Read the model definition and answer for the solid it produces. Units are mm, in the model's axes. Face numbers are marked on the shaded views. A direction names the side the tool comes from. Coordinates: 2 decimals unless noted, no trailing zeros. Write each loop counter-clockwise with the first axis right and the second up, starting at its lowest first coordinate (ties: lowest second). Pieces come first, ordered by that corner, then holes. Notation, with made-up numbers: (68.25, 57) -> (90.25, 57) arc R20 cw to (90.25, 84) -> close; hole circle Ø9 at (-0.5, -6). An arc over 180 degrees is marked (long way). Answer as a JSON object with one key per item and string values. Group by question number.
(1) Which of the six approach directions +Z, -Z, +X, -X, +Y, -Y give full straight-line access (tool end or side, diameter ignored) to the marked faces 1 and 2?
(2) A flat-ended cylindrical pin translates along its axis: P1, Ø7.5, axis at x = 0, y = 52.34, coming from the +Z side. Find the tip coordinate at first contact, or state that the pin passes through.
(3) For a pull along Z with two mould halves and no side action, classify the marked faces 3, 4 and 5 as +Z half, -Z half, draft (parallel to the pull), parting line (faces both ways), or undercut.
(4) Find section D-D (x = 1). Count the separate pieces of the cut face and the enclosed holes in it, then the cut area to 3 significant figures.
(5) Straight lines are drawn through the part: L1, parallel to Z at x = 1, y = -45.5 (3 decimals); L2, parallel to Y at x = 0, z = 11.3. For each, find the intervals that lie inside material, in ascending order.
(6) Find section A-A (x = -5.75). Give the vertices of the cut face in (y, z) (3 decimals).
(7) Find section C-C (z = -3.5). Give the vertices of the cut face in (x, y) (3 decimals).
(8) Find section B-B (y = 37.5). Give the vertices of the cut face in (x, z) (3 decimals), then the cut area to 3 significant figures.
from build123d import *

# Parameters (mm, degrees)
SKETCH1_W           = 25.4
SKETCH1_H           = 25.4
SKETCH1_W_2         = 19.05
SKETCH1_H_2         = 19.05
BOSS_EXTRUDE1_DEPTH = 82.931
CUT_EXTRUDE1_DEPTH  = 88.658432344
SKETCH3_R           = 3.22238806
CUT_EXTRUDE2_DEPTH  = 88.658432344


with BuildPart() as part:
    # Sketch1 → Boss-Extrude1 (new, symmetric)
    with BuildSketch(Plane(origin=(0, 0, 0), x_dir=(1, 0, 0), z_dir=(0, 1, 0))):
        Rectangle(SKETCH1_W, SKETCH1_H)
        Rectangle(SKETCH1_W_2, SKETCH1_H_2, mode=Mode.SUBTRACT)
    extrude(amount=BOSS_EXTRUDE1_DEPTH, both=True)

    # Sketch2 → Cut-Extrude1 (cut, through all)
    with BuildSketch(Plane(origin=(12.7, 0, 0), x_dir=(0, 0, -1), z_dir=(1, 0, 0))):
        Polygon((12.7, 82.931), (-12.7, 82.931), (12.7, 72.409975516), align=None)
        Polygon((12.7, -72.409975516), (-12.7, -82.931), (12.7, -82.931), align=None)
    extrude(amount=-CUT_EXTRUDE1_DEPTH, mode=Mode.SUBTRACT)

    # Sketch3 → Cut-Extrude2 (cut, through all)
    with BuildSketch(Plane(origin=(0, 0, -12.7), x_dir=(-1, 0, 0), z_dir=(0, 0, -1))):
        with Locations((0, -65.043975516)):
            Circle(SKETCH3_R)
        with Locations((0, -52.343975516)):
            Circle(SKETCH3_R)
        with Locations((0, 65.043975516)):
            Circle(SKETCH3_R)
        with Locations((0, 52.343975516)):
            Circle(SKETCH3_R)
    extrude(amount=-CUT_EXTRUDE2_DEPTH, mode=Mode.SUBTRACT)


solid = part.part
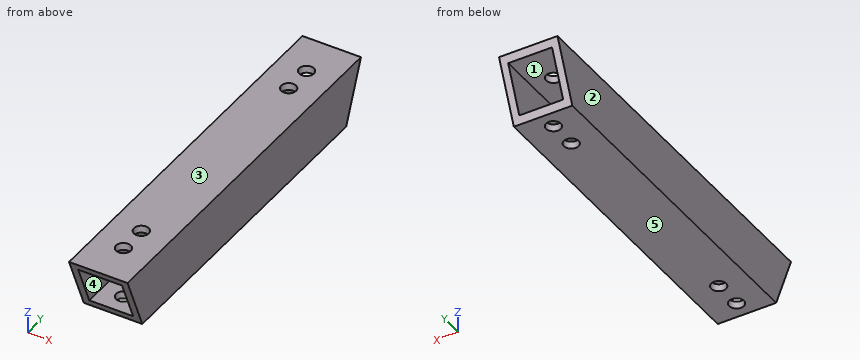
Results below:
{
 "1": {"face 1": "+Y, -Y", "face 2": "+Z, -Z, -X, +Y, -Y"},
 "2": {"P1": "stops at z = 12.7"},
 "3": {"face 3": "+Z half", "face 4": "undercut", "face 5": "-Z half"},
 "4": {"separate pieces": "10", "enclosed holes": "0", "area": "831 mm2"},
 "5": {"L1": "z = -12.7 to -9.525, 9.525 to 12.7", "L2": "y = -82.35 to -68.27, -61.82 to -55.57, -49.12 to 49.12, 55.57 to 61.82, 68.27 to 82.35"},
 "6": {"outline": "(-82.931, 12.7) -> (-81.616, 9.525) -> (81.616, 9.525) -> (82.931, 12.7) -> close; (-73.725, -9.525) -> (-72.41, -12.7) -> (72.41, -12.7) -> (73.725, -9.525) -> close"},
 "7": {"outline": "(-12.7, -76.221) -> (-9.525, -76.221) -> (-9.525, 76.221) -> (-12.7, 76.221) -> close; (9.525, -76.221) -> (12.7, -76.221) -> (12.7, 76.221) -> (9.525, 76.221) -> close"},
 "8": {"outline": "(-12.7, -12.7) -> (12.7, -12.7) -> (12.7, 12.7) -> (-12.7, 12.7) -> close; hole (-9.525, -9.525) -> (9.525, -9.525) -> (9.525, 9.525) -> (-9.525, 9.525) -> close", "area": "282 mm2"}
}
